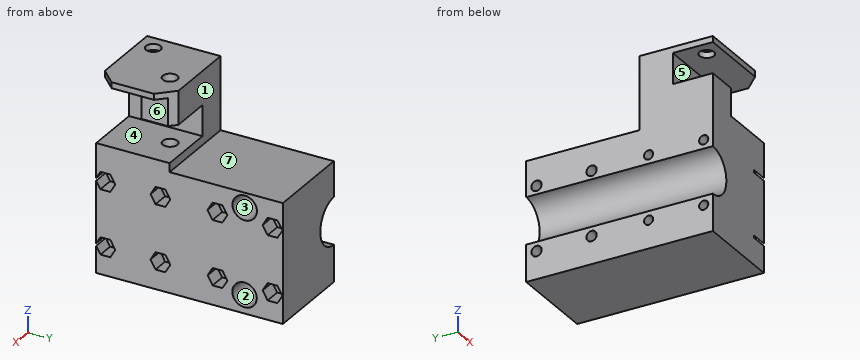
from build123d import *

# Parameters (mm, degrees)
SKETCH_W             = 28.891708
SKETCH_H             = 61.000002
PAD_DEPTH            = 64.706
POCKET_DEPTH         = 5.486
SKETCH002_R          = 4.000759
SKETCH002_R_2        = 4.000904
POCKET013_DEPTH      = 28.147
SKETCH003_R          = 7.633881
POCKET014_DEPTH      = 90
SKETCH004_R          = 1.501587
SKETCH004_R_2        = 1.6888463945
SKETCH004_R_3        = 1.688846
POCKET015_DEPTH      = 71
SKETCH005_W          = 61.94006
SKETCH005_H          = 58.87719
POCKET016_DEPTH      = 34
SKETCH006_W          = 11.564612
SKETCH006_H          = 9.981083
POCKET017_DEPTH      = 18.59
POCKET018_DEPTH      = 14
SKETCH008_W          = 13.093784
SKETCH008_H          = 9.999417
POCKET019_DEPTH      = 38
POCKET019_FACE20_W   = 18.59
POCKET019_FACE20_H   = 9.981083
POCKET020_DEPTH      = 21
SKETCH009_R          = 2.400503
POCKET021_DEPTH      = 27.202
SKETCH010_R          = 2.409031
POCKET022_DEPTH      = 27.378
SKETCH011_W          = 3.434418
SKETCH011_H          = 9.662621
POCKET023_DEPTH      = 54
POCKET023_FACE73_R   = 2.400503
POCKET023_FACE73_R_2 = 2.409031
POCKET024_DEPTH      = 2


with BuildPart() as part:
    # Sketch → Pad (new body)
    with BuildSketch(Plane.XY):
        with Locations((-167.960045, 6.499999)):
            Rectangle(SKETCH_W, SKETCH_H)
    extrude(amount=PAD_DEPTH)

    # Sketch001 (on Face2 of Pad) → Pocket (cut)
    with BuildSketch(Plane.YZ.offset(-153.514191)):
        Polygon((0.227114, 30.1176869999), (-1.3898859999, 32.9184131558), (-4.6238859999, 32.9184131559), (-6.240886, 30.1176870001), (-4.6238860001, 27.3169608442), (-1.3898860001, 27.3169608441), align=None)
        Polygon((18.864944, 30.0627266883), (17.2479442699, 32.863453), (14.0139442699, 32.8634533117), (12.396944, 30.0627273117), (14.0139437301, 27.262001), (17.2479437301, 27.2620006883), align=None)
        Polygon((36.870486, 30.0424916883), (35.2534862699, 32.843218), (32.0194862699, 32.8432183117), (30.402486, 30.0424923117), (32.0194857301, 27.241766), (35.2534857301, 27.2417656883), align=None)
        Polygon((-17.752086, 9.074409), (-19.369086, 11.8751351559), (-22.603086, 11.8751351558), (-24.220086, 9.074409), (-22.603086, 6.2736828441), (-19.369086, 6.2736828442), align=None)
        Polygon((0.225859, 9.1006766883), (-1.3911407301, 11.901403), (-4.6251407301, 11.9014033117), (-6.242141, 9.1006773117), (-4.6251412699, 6.299951), (-1.3911412699, 6.2999506883), align=None)
        Polygon((36.86032, 9.0323376883), (35.2433202699, 11.833064), (32.0093202699, 11.8330643117), (30.39232, 9.0323383117), (32.0093197301, 6.231612), (35.2433197301, 6.2316116883), align=None)
        Polygon((18.890709, 9.0329989998), (17.2737090002, 11.8337251557), (14.0397090002, 11.8337251559), (12.422709, 9.0329990002), (14.0397089998, 6.2322728443), (17.2737089998, 6.2322728441), align=None)
        Polygon((-17.770354, 30.0952738442), (-19.387354, 32.896), (-22.621354, 32.896), (-24.238354, 30.0952738442), (-22.621354, 27.2945476883), (-19.387354, 27.2945476883), align=None)
    extrude(amount=-POCKET_DEPTH, mode=Mode.SUBTRACT)

    # Sketch002 (on Face3 of Pocket) → Pocket013 (cut)
    with BuildSketch(Plane.YZ.offset(-153.514191)):
        with Locations((24.525928, 33.978888)):
            Circle(SKETCH002_R)
        with Locations((24.483081, 5.987167)):
            Circle(SKETCH002_R_2)
    extrude(amount=-POCKET013_DEPTH, mode=Mode.SUBTRACT)

    # Sketch003 (on Face1 of Pocket013) → Pocket014 (cut)
    with BuildSketch(Plane.XZ.offset(24.000002)):
        with Locations((-182.392539, 19.658504)):
            Circle(SKETCH003_R)
    extrude(amount=-POCKET014_DEPTH, mode=Mode.SUBTRACT)

    # Sketch004 (on Face3 of Pocket014) → Pocket015 (cut)
    with BuildSketch(Plane.YZ.offset(-153.514191)):
        with Locations((-2.992992, 30.128542)):
            Circle(SKETCH004_R)
        with Locations((15.650433, 9.031955)):
            Circle(SKETCH004_R_2)
        with Locations((-21.003469, 9.112989)):
            Circle(SKETCH004_R)
        with Locations((-3.007213, 9.130702)):
            Circle(SKETCH004_R)
        with Locations((-21.01451, 30.1173)):
            Circle(SKETCH004_R)
        with Locations((33.645615, 30.049736)):
            Circle(SKETCH004_R_3)
        with Locations((33.606518, 9.031116)):
            Circle(SKETCH004_R_3)
        with Locations((15.625216, 30.036369)):
            Circle(SKETCH004_R_3)
    extrude(amount=-POCKET015_DEPTH, mode=Mode.SUBTRACT)

    # Sketch005 (on Face3 of Pocket015) → Pocket016 (cut)
    with BuildSketch(Plane.YZ.offset(-153.514191)):
        with Locations((30.97003, 68.319813)):
            Rectangle(SKETCH005_W, SKETCH005_H)
    extrude(amount=-POCKET016_DEPTH, mode=Mode.SUBTRACT)

    # Sketch006 (on Face3 of Pocket016) → Pocket017 (cut)
    with BuildSketch(Plane.YZ.offset(-153.514191)):
        with Locations((-5.122813, 46.7572385)):
            Rectangle(SKETCH006_W, SKETCH006_H)
    extrude(amount=-POCKET017_DEPTH, mode=Mode.SUBTRACT)

    # Sketch007 (on Face10 of Pocket017) → Pocket018 (cut)
    with BuildSketch(Plane.XY.offset(64.706)):
        Polygon((-158.429092, -23.970312), (-153.252335, -18.703115), (-151.097504, -28.69935), align=None)
        Polygon((-153.520828, -5.084184), (-159.130096, 0.622078), (-148.158478, 1.033419), align=None)
    extrude(amount=-POCKET018_DEPTH, mode=Mode.SUBTRACT)

    # Sketch008 (on Face13 of Pocket018) → Pocket019 (cut)
    with BuildSketch(Plane(origin=(-182.405899, 0, 0), x_dir=(0, -1, 0), z_dir=(-1, 0, 0))):
        with Locations((17.453488, 55.7602025)):
            Rectangle(SKETCH008_W, SKETCH008_H)
    extrude(amount=-POCKET019_DEPTH, mode=Mode.SUBTRACT)

    # Pocket019 Face20 → Pocket020 (cut)
    with BuildSketch(Plane(origin=(-162.809191, -10.905119, 46.7572385), x_dir=(1, 0, 0), z_dir=(0, 1, 0))):
        Rectangle(POCKET019_FACE20_W, POCKET019_FACE20_H)
    extrude(amount=-POCKET020_DEPTH, mode=Mode.SUBTRACT)

    # Sketch009 (on Face68 of Pocket020) → Pocket021 (cut)
    with BuildSketch(Plane.XY.offset(64.706)):
        with Locations((-177.111391, -18.947801)):
            Circle(SKETCH009_R)
    extrude(amount=-POCKET021_DEPTH, mode=Mode.SUBTRACT)

    # Sketch010 (on Face72 of Pocket021) → Pocket022 (cut)
    with BuildSketch(Plane.XY.offset(64.706)):
        with Locations((-164.116726, -5.948229)):
            Circle(SKETCH010_R)
    extrude(amount=-POCKET022_DEPTH, mode=Mode.SUBTRACT)

    # Sketch011 (on Face1 of Pocket022) → Pocket023 (cut)
    with BuildSketch(Plane.XZ.offset(24.000002)):
        with Locations((-154.641205, 55.9206505)):
            Rectangle(SKETCH011_W, SKETCH011_H)
    extrude(amount=-POCKET023_DEPTH, mode=Mode.SUBTRACT)

    # Pocket023 Face73 → Pocket024 (cut)
    with BuildSketch(Plane(origin=(-168.318188921, -11.9801298357, 64.706), x_dir=(0, 1, 0), z_dir=(0, 0, 1))):
        Polygon((11.9801298357, -9.7995969527), (11.9801298357, 14.087710079), (-12.0198721643, 14.087710079), (-12.0198721643, -9.935126335), (-11.9901821643, -9.889096921), (-6.9894158925, -14.803997921), (6.9035176151, -14.803997921), (6.8959458357, -14.797360921), align=None)
        with Locations((-6.9676711643, 8.793202079)):
            Circle(POCKET023_FACE73_R, mode=Mode.SUBTRACT)
        with Locations((6.0319008357, -4.201462921)):
            Circle(POCKET023_FACE73_R_2, mode=Mode.SUBTRACT)
    extrude(amount=-POCKET024_DEPTH, mode=Mode.SUBTRACT)


solid = part.part
The listing builds one solid part. Answer for the finished solid, in the listing's coordinates (mm). Face numbers are marked on the shaded views. A direction names the side the tool comes from. Coordinates: 2 decimals unless noted, no trailing zeros. Loops run counter-clockwise (first coordinate to the right, second up) from the corner with the lowest first, then second, coordinate; pieces in that order, holes last. Notation, with made-up numbers: M 6.5,73 L 60.5,73 A10 cw 60.5,86 Z; hole C 24.25,-5.5 d9. An arc over 180 degrees is marked long. Answer in a Markdown table with one row per item.
1) Find section C-C (y = 2). Determine the outline of the cut face in (x, z), then the cut area to 3 significant figures.
Answers below:
| item | result |
|---|---|
| outline | M -182.41,0 L -153.51,0 L -153.51,38.88 L -182.41,38.88 L -182.41,27.29 A7.63 cw -182.41,12.02 Z |
| area | 1,030 mm^2 |
2) Given pin 1 (10 mm diameter, centred on x = -157, z = 48, fed in from -Y); pin 2 (7.5 mm diameter, centred on x = -164.12, y = -5.95, fed in from +Z); pin 3 (2.5 mm diameter, centred on x = -155, y = 15.5, fed in from +Z); pin 4 (3.5 mm diameter, centred on y = -3.01, z = 9.13, fed in from +X), each flat-ended and moving along its own axis, determine where each tip first touches the part or whether it passes through.
Answers below:
| item | result |
|---|---|
| pin 1 | y = -10.91 |
| pin 2 | z = 62.71 |
| pin 3 | z = 38.88 |
| pin 4 | x = -159 |
3) Determine the mould class of the marked faces 1, 2, 3 and 4 for opening direction Y: released by +Y, released by -Y, zero draft, split by the parting line, or undercut.
Answers below:
| item | result |
|---|---|
| face 1 | released by +Y |
| face 2 | undercut |
| face 3 | undercut |
| face 4 | zero draft |
4) Find the intervals of material crossed by probe 1 along Z at (x, y) = (-179.5, 23); probe 2 along Z at (x, y) = (-168.5, -15.5); probe 3 along X at (y, z) = (-6, 58), in increasing order.
Answers below:
| item | result |
|---|---|
| probe 1 | 0 to 2.27, 9.7 to 12.59, 26.72 to 30.28, 37.68 to 38.88 |
| probe 2 | 0 to 41.77, 60.76 to 62.71 |
| probe 3 | -182.41 to -166.53, -161.71 to -156.36 |
5) Find section A-A (y = -15). Determine the outline of the cut face in (x, z).
Answers below:
| item | result |
|---|---|
| outline | M -182.41,0 L -153.51,0 L -153.51,41.77 L -172.1,41.77 L -172.1,50.76 L -182.41,50.76 L -182.41,27.29 A7.63 cw -182.41,12.02 Z; M -182.41,60.76 L -153.51,60.76 L -153.51,62.71 L -182.41,62.71 Z |
6) Which of the six approach directions +Z, -Z, +X, -X, +Y, -Y give full straight-line access (tool end or side, diameter ignored) to the marked faces 5, 6 and 7?
Answers below:
| item | result |
|---|---|
| face 5 | +X, -X, -Y |
| face 6 | +X, +Y, -Y |
| face 7 | +Z, +X, -X, +Y |
7) Find section B-B (z = 54). Determine the outline of the cut face in (x, y).
Answers below:
| item | result |
|---|---|
| outline | M -182.41,-10.91 L -156.36,-10.91 L -156.36,-2.2 L -158.52,0 L -182.41,0 Z; hole C -164.12,-5.95 d4.82 |
